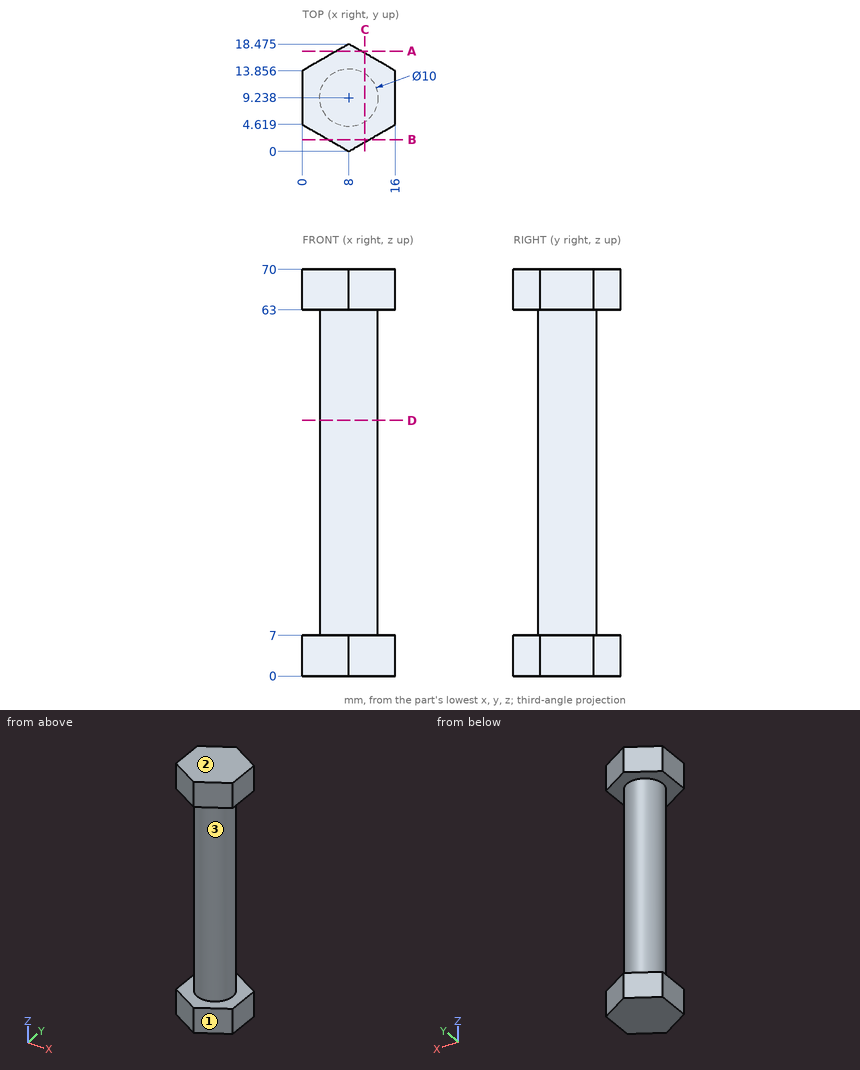
Source: three-view drawing plus pictorial views. Frame: mm from the lowest corner of the part. Round coordinates to 2 decimals unless told otherwise and drop trailing zeros. Write each loop counter-clockwise with the first axis right and the second up, starting at its lowest first coordinate (ties: lowest second). Pieces come first, ordered by that corner, then holes. Notation, with made-up numbers: M 79.25,65 L 125.25,65 A17 cw 125.25,90 Z; hole C -15.75,-11 d3. An arc over 180 degrees is marked long. Write item = value, one per line.
Item 1: Pull-direction query (Z, two-part tool) for the marked faces 1, 2 and 3; classes: pulls with the +Z half, pulls with the -Z half, needs draft (parallel to the pull), parting line crosses it, or undercut.
Findings:
face_1 = needs draft
face_2 = pulls with the +Z half
face_3 = undercut
Item 2: Section query D-D on z = 44. Return loops of the section in (x, y).
Findings:
outline = C 8,9.24 d10
Item 3: Material intervals for line 1 along Z through (x, y) = (12.5, 15.5); line 2 along Y through (x, z) = (11.25, 3.5) (1 decimal); line 3 along Y through (x, z) = (6.5, 19.5), sorted ascending. Write a range as [from, to].
Findings:
line_1 = [0, 7], [63, 70]
line_2 = [1.9, 16.6]
line_3 = [4.47, 14.01]
Item 4: Section query B-B on y = 2. Return loops of the section in (x, z).
Findings:
outline = M 4.54,0 L 11.46,0 L 11.46,7 L 4.54,7 Z; M 4.54,63 L 11.46,63 L 11.46,70 L 4.54,70 Z
Item 5: Section query A-A on y = 17.25. Return loops of the section in (x, z).
Findings:
outline = M 5.88,0 L 10.12,0 L 10.12,7 L 5.88,7 Z; M 5.88,63 L 10.12,63 L 10.12,70 L 5.88,70 Z
Item 6: Section query C-C on x = 10.75. Return loops of the section in (y, z), then the cut area to 3 significant figures.
Findings:
outline = M 1.59,0 L 16.89,0 L 16.89,7 L 13.41,7 L 13.41,63 L 16.89,63 L 16.89,70 L 1.59,70 L 1.59,63 L 5.06,63 L 5.06,7 L 1.59,7 Z
area = 682 mm^2
Item 7: Pin query (flat end, axial travel): P1, Ø3, axis at x = 11, z = 15, coming from the -Y side; P2, Ø6, axis at y = 15, z = 24.5, coming from the -X side; P3, Ø4, axis at x = 12, z = 11, coming from the -Y side (1 decimal). Return the tip coordinate at first contact, or that it passes through.
Findings:
P1 = 4.47
P2 = 3.83
P3 = 4.7
